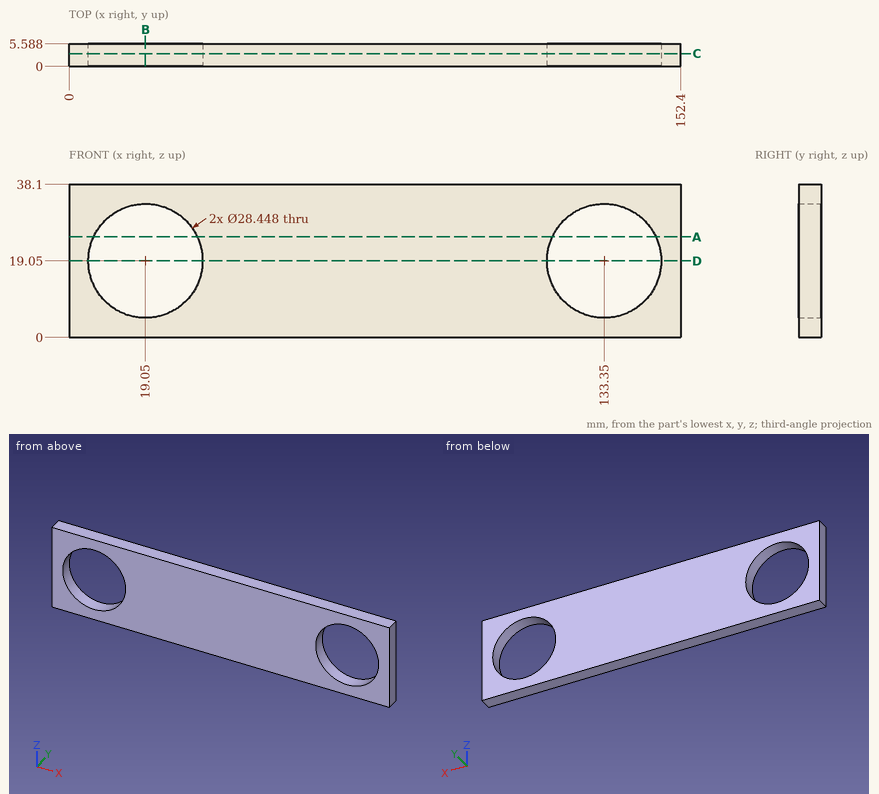
Job drawing, mm, ordinate dimensions from the low corner. One solid piece. Round coordinates to 2 decimals unless told otherwise and drop trailing zeros. Loops run counter-clockwise (first coordinate to the right, second up) from the corner with the lowest first, then second, coordinate; pieces in that order, holes last. Notation, with made-up numbers: M 61.5,44.5 L 75.5,44.5 A19 cw 75.5,57.5 Z; hole C 40.25,-39 d5. An arc over 180 degrees is marked long. One line per question, with ' | ' between items. Start each with the question number.
Item 1: Cut at A-A, the plane z = 25. Write the cut outline in (x, y).
Item 2: Cut at B-B, the plane x = 19.05. Write the cut outline in (y, z), plus the area to 3 significant figures.
Item 3: Cut at C-C, the plane y = 3.2. Write the cut outline in (x, z).
Item 4: Wall check: line 1 (X direction, y = 3.4, z = 19.05); line 2 (Z direction, x = 133.35, y = 1.8); line 3 (X direction, y = 4.05, z = 21). Give the ranges that are in metal, low to high.
Item 5: Cut at D-D, the plane z = 19.05. Write the cut outline in (x, y), plus the area to 3 significant figures.
Item 6: Pin check, flat tip, straight feed: pin 1 Ø1.5 at (x, y) = (91, 3) entering from -Z. Stop position of the tip, or through.
Responses:
1) outline: M 0,0 L 6.13,0 L 6.13,5.59 L 0,5.59 Z; M 31.97,0 L 120.43,0 L 120.43,5.59 L 31.97,5.59 Z; M 146.27,0 L 152.4,0 L 152.4,5.59 L 146.27,5.59 Z
2) outline: M 0,0 L 5.59,0 L 5.59,4.83 L 0,4.83 Z; M 0,33.27 L 5.59,33.27 L 5.59,38.1 L 0,38.1 Z | area: 53.9 mm²
3) outline: M 0,0 L 152.4,0 L 152.4,38.1 L 0,38.1 Z; hole C 19.05,19.05 d28.45; hole C 133.35,19.05 d28.45
4) line 1: x = 0 to 4.83, 33.27 to 119.13, 147.57 to 152.4 | line 2: z = 0 to 4.83, 33.27 to 38.1 | line 3: x = 0 to 4.96, 33.14 to 119.26, 147.44 to 152.4
5) outline: M 0,0 L 4.83,0 L 4.83,5.59 L 0,5.59 Z; M 33.27,0 L 119.13,0 L 119.13,5.59 L 33.27,5.59 Z; M 147.57,0 L 152.4,0 L 152.4,5.59 L 147.57,5.59 Z | area: 534 mm²
6) pin 1: stops at z = 0
